```python
from build123d import *

# Parameters (mm, degrees)
F1_DEPTH = 1.5
F3_DEPTH = 0.5
F5_DEPTH = 0.5
F7_DEPTH = 3


# Not quite as in the source:
# - ends of sketch curves that miss each other by under 0.0002 mm in the source are joined
# - a feature names something its author has since deleted; it is built from what else it names


with BuildPart() as f1:
    # F0 (on Front) → F1 (new body, symmetric)
    with BuildSketch(Plane.XZ):
        Polygon((0, 40), (0, 0), (5, 0), (5, 15), (3.7145695426, 16.5003631264), (3.7145695426, 21.137110889), (2.2125243451, 22.1820119768), (3.7145695426, 24.5330389589), (3.7145695426, 26.7870686948), (1.7496975381, 26.7870686948), (1.7496975381, 27.8878770769), (3.7145695426, 28.8214460015), (3.7266683541, 30.0295948982), (2.903013601, 30.0378432554), (2.903013601, 31.4024910331), (3.7145695426, 31.4024910331), (3.7145695426, 34.1644659638), (1.2732772157, 39.1865172364), align=None)
        Polygon((-1.2732772157, 0), (0, 0), (0, 40), (-1.2732772157, 39.1865172364), align=None)
        Polygon((-5, 0), (-1.2732772157, 0), (-1.2732772157, 39.1865172364), (-3.7145695426, 34.1644659638), (-3.7145695426, 31.4024910331), (-2.903013601, 31.4024910331), (-2.903013601, 30.0378432554), (-3.7266683541, 30.0295948982), (-3.7145695426, 28.8214460015), (-1.7496975381, 27.8878770769), (-1.7496975381, 26.7870686948), (-3.7145695426, 26.7870686948), (-3.7145695426, 24.5330389589), (-2.2125243451, 22.1820119768), (-3.7145695426, 21.137110889), (-3.7145695426, 16.5003631264), (-5, 15), align=None)
    extrude(amount=F1_DEPTH, both=True)

    # F2 (on face) → F3 (cut)
    with BuildSketch(Plane.XZ.offset(1.5)):
        Polygon((0, 0), (0, 40), (-1.2732772157, 39.1865172364), (-1.2732772157, 0), align=None)
    extrude(amount=-F3_DEPTH, mode=Mode.SUBTRACT)

    # F4 (on face) → F5 (cut)
    with BuildSketch(Plane(origin=(0, 1.5, 0), x_dir=(-1, 0, 0), z_dir=(0, 1, 0))):
        Polygon((1.2732772157, 0), (1.2732772157, 39.1865172364), (0, 40), (0, 0), align=None)
    extrude(amount=-F5_DEPTH, mode=Mode.SUBTRACT)

    # F6 (on face) → F7 (join)
    with BuildSketch(Plane(origin=(0, 1.5, 0), x_dir=(-1, 0, 0), z_dir=(0, 1, 0))):
        with BuildLine():
            Line((-5, 0), (-4.9999982459, -4.1340150831))
            ThreePointArc((-4.9999982459, -4.1340150831), (-3.5355314017, -7.6695476176), (1.7541e-06, -9.1340129616))
            Line((1.7541e-06, -9.1340129616), (1.3932e-06, -6.5670064808))
            ThreePointArc((1.3932e-06, -6.5670064808), (-1.9999990311, -4.5670062085), (5.446e-07, -2.5670064808))
            Line((5.446e-07, -2.5670064808), (0, 0))
            Line((0, 0), (-5, 0))
        make_face()
        with BuildLine():
            Line((1.3932e-06, -6.5670064808), (1.9378e-06, -9.1340129616))
            ThreePointArc((1.9378e-06, -9.1340129616), (3.5355339059, -7.6695468675), (5, -4.1340129616))
            Line((5, -4.1340129616), (5, 0))
            Line((5, 0), (0, 0))
            Line((0, 0), (5.446e-07, -2.5670064808))
            ThreePointArc((5.446e-07, -2.5670064808), (1.4142143813, -3.1527927684), (2.0000009689, -4.5670064808))
            ThreePointArc((2.0000009689, -4.5670064808), (1.4142141887, -5.9812203857), (1.3932e-06, -6.5670064808))
        make_face()
    extrude(amount=-F7_DEPTH)


solid = f1.part
```
Here's how the part is built. I have some questions about the finished solid (model axes, mm). A direction names the side the tool comes from. Coordinates: 2 decimals unless noted, no trailing zeros. Loops run counter-clockwise (first coordinate to the right, second up) from the corner with the lowest first, then second, coordinate; pieces in that order, holes last. Notation, with made-up numbers: M 25,-13.5 L 46,-13.5 A15 cw 46,3.5 Z; hole C 84,87 d6. An arc over 180 degrees is marked long. One line per item, written item: value.
1. On a 3-axis mill with a long thin cutter (end or side, diameter ignored), from which of +Z, -Z, +X, -X, +Y, -Y can I reach the whole of each face in a straight line? I mean faces 5 (the flat face through (-2.95, -0.02, 21.67)), 6 (the flat face through (1.75, 0, 27)). Say none if no direction works.
Geometry says:
face 5: -X, +Y, -Y
face 6: +X, +Y, -Y
2. Please list where these lines run through material, in increasing order: probe 1 along X at (y, z) = (1.25, 1); probe 2 along Z at (x, y) = (2.75, 1); probe 3 along Z at (x, y) = (-2.5, 0).
Geometry says:
probe 1: x = -5 to -1.27, 0 to 5
probe 2: z = -8.31 to 21.81, 23.02 to 26.79, 28.36 to 36.15
probe 3: z = -8.46 to 21.98, 22.63 to 26.79, 28.24 to 36.66
3. Will these pins go through, and if not, where does the flat tip stop? pin 1 Ø0.7 at (y, z) = (0, 31) entering from +X; pin 2 Ø1.6 at (x, y) = (2.5, 0.5) entering from +Z; pin 3 Ø0.6 at (y, z) = (1, 23) entering from -X.
Geometry says:
pin 1: stops at x = 2.9
pin 2: stops at z = 38.31
pin 3: stops at x = -2.93
4. Imagine slicing it at A-A (x = 4.5). List the corners of the cut face in (y, z) for me, and give its area (3 significant figures).
Geometry says:
outline: M -1.5,-6.31 L 1.5,-6.31 L 1.5,15.58 L -1.5,15.58 Z
area: 65.7 mm2
5. Thinking about a two-plate mould opening in Z: for faces 1 (the flat face through (-3, 0, 26.787)), 2 (the flat face through (3.3, 0, 31.402)), 3 (the flat face through (0.646, -0.021, 39.588)), 4 (the flat face through (-1, 1, 20)), which applies, +Z half, -Z half, draft (parallel to the pull), parting line (faces both ways), or undercut?
Geometry says:
face 1: undercut
face 2: undercut
face 3: +Z half
face 4: draft
